```python
from build123d import *

# Parameters (mm, degrees)
F0_R     = 5.588
F0_R_2   = 3.937
F0_R_3   = 2.286
F1_DEPTH = 2.413
F2_DEPTH = 0.762
F3_SIZE  = 0.3


with BuildPart() as f1:
    # F0 (on Front) → F1 (new body, symmetric)
    with BuildSketch(Plane.XZ):
        Circle(F0_R)
        Circle(F0_R_2, mode=Mode.SUBTRACT)
        Circle(F0_R_2)
        Circle(F0_R_3, mode=Mode.SUBTRACT)
    extrude(amount=F1_DEPTH, both=True)

    # F0 (on Front) → F2 (cut, symmetric)
    with BuildSketch(Plane.XZ):
        Circle(F0_R)
        Circle(F0_R_2, mode=Mode.SUBTRACT)
    extrude(amount=F2_DEPTH, both=True, mode=Mode.SUBTRACT)

    # F3
    f3_edges = [f1.edges().sort_by_distance(p)[0] for p in [
        (-2.286, -2.413, 0),
        (-2.286, 2.413, 0),
    ]]
    chamfer(f3_edges, length=F3_SIZE)


solid = f1.part
```
Geometry check sheet. Reference: the model listing, model coordinates, mm. A direction names the side the tool comes from. Coordinates: 2 decimals unless noted, no trailing zeros. Order: outer loops, then holes, each group sorted by start corner. A loop starts at its lowest first (then second) coordinate and runs counter-clockwise, first axis right, second up.
Q1. Sectioned sample at D-D on y = -1.2. Record the cut outline in (x, z), and give its area (3 significant figures).
Reply:
outline: circle Ø11.18 at (0, 0); hole circle Ø4.57 at (0, 0)
area: 81.7 mm2
Q2. Tool access check on faces 4 (the face through (-4.434, 1.576, -3.4)), 5 (the face through (-0.853, 0.011, -3.843)). Record the directions out of +Z, -Z, +X, -X, +Y, -Y that give a thin tool (end or side, any length) a straight path to the whole face; none if there is none.
Reply:
face 4: +Y, -Y
face 5: none
Q3. Draft check along Z on faces 1 (the face through (-4.434, -1.599, -3.4)), 2 (the face through (2.41, -2.413, 1.32)), 3 (the face through (-0.5, 0.03, -2.23)). Enter one of: released by +Z, released by -Z, zero draft, split by the parting line, or undercut.
Reply:
face 1: split by the parting line
face 2: zero draft
face 3: undercut
Q4. Sectioned sample at A-A on x = 0. Record the cut outline in (y, z).
Reply:
outline: (-2.41, -5.59) - (-0.76, -5.59) - (-0.76, -3.94) - (0.76, -3.94) - (0.76, -5.59) - (2.41, -5.59) - (2.41, -2.59) - (2.11, -2.29) - (-2.11, -2.29) - (-2.41, -2.59) - close; (-2.41, 2.59) - (-2.11, 2.29) - (2.11, 2.29) - (2.41, 2.59) - (2.41, 5.59) - (0.76, 5.59) - (0.76, 3.94) - (-0.76, 3.94) - (-0.76, 5.59) - (-2.41, 5.59) - close
Q5. Sectioned sample at C-C on y = -0.35. Record the cut outline in (x, z), and give its area (3 significant figures).
Reply:
outline: circle Ø7.87 at (0, 0); hole circle Ø4.57 at (0, 0)
area: 32.3 mm2
Q6. Sectioned sample at B-B on z = 0. Record the cut outline in (x, y), and give its area (3 significant figures).
Reply:
outline: (-5.59, -2.41) - (-2.59, -2.41) - (-2.29, -2.11) - (-2.29, 2.11) - (-2.59, 2.41) - (-5.59, 2.41) - (-5.59, 0.76) - (-3.94, 0.76) - (-3.94, -0.76) - (-5.59, -0.76) - close; (2.29, -2.11) - (2.59, -2.41) - (5.59, -2.41) - (5.59, -0.76) - (3.94, -0.76) - (3.94, 0.76) - (5.59, 0.76) - (5.59, 2.41) - (2.59, 2.41) - (2.29, 2.11) - close
area: 26.7 mm2
Q7. Depth check by flat-ended pin: pin 1 Ø1 at (y, z) = (1.5, -3.5) entering from +X; pin 2 Ø1.5 at (x, y) = (-2, 1.5) entering from +Z. Enter the tip coordinate at first touch or a pass-through.
Reply:
pin 1: stops at x = 4.71
pin 2: stops at z = 5.45
Q8. Thickness scan on probe 1 along Y at (x, z) = (4.25, 0.5); probe 2 along Z at (x, y) = (0, 1.35); probe 3 along X at (y, z) = (0.6, -2). Record the ranges inside material, lowest first.
Reply:
probe 1: y = -2.41 to -0.76, 0.76 to 2.41
probe 2: z = -5.59 to -2.29, 2.29 to 5.59
probe 3: x = -3.39 to -1.11, 1.11 to 3.39
